The model under review builds one solid part; all positions refer to its coordinate system, in mm. Face numbers are marked on the shaded views. A direction names the side the tool comes from. Round coordinates to 2 decimals unless told otherwise and drop trailing zeros. Write each loop counter-clockwise with the first axis right and the second up, starting at its lowest first coordinate (ties: lowest second). Pieces come first, ordered by that corner, then holes.
Item 1: Add section A-A (y = 0). Give the boundary of the cut face in (x, z), plus the area to 3 significant figures.
Item 2: Add section D-D (x = 9). Give the boundary of the cut face in (y, z).
Item 3: To check wall thickness, follow L1, parallel to Z at x = -0.5, y = 3; L2, parallel to Y at x = 43, z = -5.75; L3, parallel to X at y = 0, z = -0.5. State the ranges of each line that lie inside material, in increasing order.
Item 4: Add section C-C (x = 18.5). Give the boundary of the cut face in (y, z).
Item 5: Add section B-B (z = 0). Give the boundary of the cut face in (x, y), plus the area to 3 significant figures.
Item 6: Draft analysis for pull direction X (two halves, no side actions). For the marked faces 1, 2, 3 and 4, state which applies: +X half, -X half, draft (parallel to the pull), parting line (faces both ways), or undercut.
Item 7: Clearance check with flat-ended pins moving along their axes: pin 1 Ø12 at (y, z) = (0.5, 6) entering from +X; pin 2 Ø1.5 at (y, z) = (14, -7) entering from +X; pin 3 Ø6 at (x, z) = (-2.5, 1.5) entering from -Y; pin 4 Ø4 at (x, y) = (24, -15) entering from -Z. State where each tip first meets the part, or that it passes through.
Item 8: Machinability: for the marked faces 5 and 6, which of the approach directions +Z, -Z, +X, -X, +Y, -Y give a long, thin tool a straight path to every point of the face, cutting with its end or side? Answer none if there is none.
```python
from build123d import *

# Parameters (mm, degrees)
F0_W          = 2.5
F0_H          = 20
F1_ANGLE_BACK = 105
F1_ANGLE      = 210
F2_DEPTH      = 4
F4_D          = 9
F5_R          = 2
F6_R          = 5
F7_R          = 5


# Not quite as in the source:
# - a feature names something its author has since deleted; it is built from what else it names


with BuildPart() as f1:
    # F0 (on Front) → F1 (revolve)
    with BuildSketch(Plane.XZ, mode=Mode.PRIVATE) as f1_sk:
        with Locations((16.0981313139, 0)):
            Rectangle(F0_W, F0_H)
    revolve(f1_sk.sketch.rotate(Axis((42.8481313139, 0, -3.3182863891), (0, 0, -1)), -F1_ANGLE_BACK), axis=Axis((42.8481313139, 0, -3.3182863891), (0, 0, -1)), revolution_arc=F1_ANGLE)

    # F0 (on Front) → F2 (join, symmetric)
    with BuildSketch(Plane.XZ):
        Polygon((14.8481313139, -10), (14.8481313139, 10), (-0.1518686861, 10), (-8.1518686861, 10), (-8.1518686861, -1.747650138), (-8.1518686861, -10), (-0.1518686861, -10), align=None)
        with Locations((16.0981313139, 0)):
            Rectangle(F0_W, F0_H)
    extrude(amount=F2_DEPTH, both=True)

    # F4 (through all)
    with Locations(Plane.XZ.offset(4)):
        with Locations((-0.1518686861, 0)):
            Hole(F4_D / 2)

    # F5
    f5_edges = [f1.edges().sort_by_distance(p)[0] for p in [
        (15.135318, -4, 0),
        (15.135318, 4, 0),
    ]]
    fillet(f5_edges, radius=F5_R)

    # F6
    f6_edges = [f1.edges().sort_by_distance(p)[0] for p in [
        (49.771541, -25.838516, 10),
        (49.771541, -25.838516, -10),
        (49.771541, 25.838516, -10),
        (49.771541, 25.838516, 10),
    ]]
    fillet(f6_edges, radius=F6_R)

    # F7
    f7_edges = [f1.edges().sort_by_distance(p)[0] for p in [
        (-8.151869, 0, 10),
        (-8.151869, 0, -10),
    ]]
    fillet(f7_edges, radius=F7_R)


solid = f1.part
```
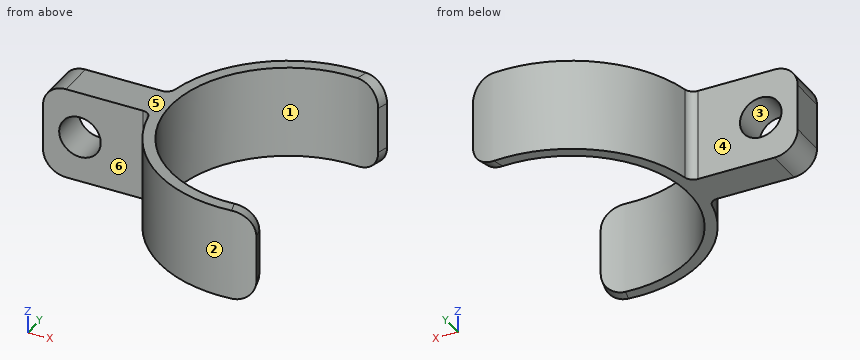
Numbers:
1. outline: (-8.15, -5) arc R5 ccw to (-3.15, -10) - (17.35, -10) - (17.35, 10) - (-3.15, 10) arc R5 ccw to (-8.15, 5) - close; hole circle Ø9 at (-0.15, 0)
1. area: 436 mm2
2. outline: (-4, -10) - (4, -10) - (4, 10) - (-4, 10) - close
3. L1: z = -10 to -4.49, 4.49 to 10
3. L2: y = -28 to -25.5, 25.5 to 28
3. L3: x = -8.15 to -4.62, 4.32 to 17.35
4. outline: (-13.83, -10) - (-7.58, -10) - (-7.58, 10) - (-13.83, 10) - close; (7.58, -10) - (13.83, -10) - (13.83, 10) - (7.58, 10) - close
5. outline: (-8.15, -4) - (-4.65, -4) - (-4.65, 4) - (-8.15, 4) - close; (4.35, -4) - (13.45, -4) arc R2 cw to (15.41, -5.6) arc R28 ccw to (50.1, -27.05) - (49.45, -24.63) arc R25.5 cw (long way) to (49.45, 24.63) - (50.1, 27.05) arc R28 ccw to (15.41, 5.6) arc R2 cw to (13.45, 4) - (4.35, 4) - close
5. area: 359 mm2
6. face 1: undercut
6. face 2: parting line
6. face 3: undercut
6. face 4: draft
7. pin 1: stops at x = 18.19
7. pin 2: stops at x = 22.05
7. pin 3: stops at y = -4
7. pin 4: stops at z = -10
8. face 5: +Z, +X, -X, +Y, -Y
8. face 6: +Z, -Z, -X, -Y
